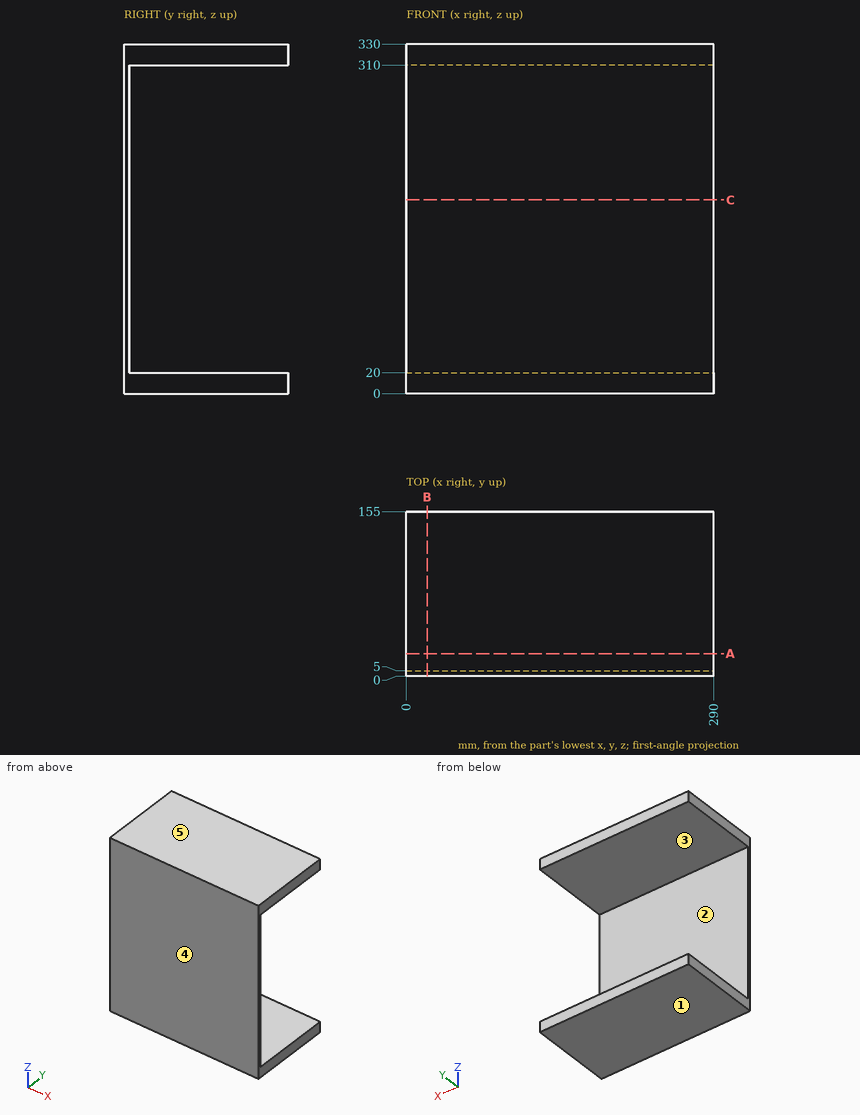
Geometry check sheet. Reference: drawing and pictorial views, mm from the part's lowest x, y, z. A direction names the side the tool comes from. Round coordinates to 2 decimals unless told otherwise and drop trailing zeros. Loops run counter-clockwise (first coordinate to the right, second up) from the corner with the lowest first, then second, coordinate; pieces in that order, holes last. Notation, with made-up numbers: (-8, 50.25) - (31, 50.25) arc R20 cw to (31, 85.25) - close; hole circle Ø9 at (25, 33). An arc over 180 degrees is marked (long way). Write item = value, one per line. Start each with the question number.
Q1. Section check B-B (x = 19.5). Record the boundary of the cut face in (y, z), plus the area to 3 significant figures.
Q2. Section check C-C (z = 183). Record the boundary of the cut face in (x, y).
Q3. Release check for a two-part mould opening along Z. For the marked faces 3, 4 and 5 record: pulls with the +Z half, pulls with the -Z half, needs draft (parallel to the pull), parting line crosses it, or undercut.
Q4. Access from +Z, -Z, +X, -X, +Y, -Y to the whole of each face (thin tool, end or side, straight path). Record for the marked faces 1 and 2.
Q5. Section check A-A (y = 21). Record the boundary of the cut face in (x, z).
Q6. Thickness scan on L1, parallel to Z at x = 135.5, y = 44; L2, parallel to Y at x = 55.5, z = 202. Record the ranges inside material, lowest first.
Derived:
q1.outline = (0, 0) - (155, 0) - (155, 20) - (5, 20) - (5, 310) - (155, 310) - (155, 330) - (0, 330) - close
q1.area = 7,650 mm^2
q2.outline = (0, 0) - (290, 0) - (290, 5) - (0, 5) - close
q3.face_3 = undercut
q3.face_4 = needs draft
q3.face_5 = pulls with the +Z half
q4.face_1 = -Z, +X, -X, +Y, -Y
q4.face_2 = +X, -X, +Y
q5.outline = (0, 0) - (290, 0) - (290, 20) - (0, 20) - close; (0, 310) - (290, 310) - (290, 330) - (0, 330) - close
q6.L1 = 0 to 20, 310 to 330
q6.L2 = 0 to 5
